Geometry check sheet. Reference: the model listing, model coordinates, mm. A direction names the side the tool comes from. Give positions to 0.01 mm unless a question says otherwise; leave off trailing zeros. Write each loop counter-clockwise with the first axis right and the second up, starting at its lowest first coordinate (ties: lowest second). Pieces come first, ordered by that corner, then holes. Notation, with made-up numbers: M 3.25,-6.75 L 48.25,-6.75 A34 cw 48.25,31.25 Z; hole C 54,-2.75 d6. An arc over 180 degrees is marked long. One line per item, written item: value. Start each with the question number.
1. Cross-section at B-B on z = 0. Record the cut outline in (x, y), then the cut area to 3 significant figures.
2. Gauge pin test, flat ends, axial feed: pin 1 (3 mm diameter, centred on y = 11, z = -22, fed in from +X); pin 2 (1 mm diameter, centred on y = 23, z = -7.5, fed in from +X); pin 3 (10 mm diameter, centred on y = 5, z = -12, fed in from -X). Record the tip position at first contact, or that the pin passes through.
3. Tool access check on faces 1 (the face through (-0.028, 17.255, 32.946)), 2 (the face through (-26.288, 21.514, 14.966)). Record the directions out of +Z, -Z, +X, -X, +Y, -Y that give a thin tool (end or side, any length) a straight path to the whole face; none if there is none.
4. Release check for a two-part mould opening along Z. For faces 3 (the face through (27.5, 21.5, 0.1)), 4 (the face through (0, 17, -33)), 5 (the face through (28, 35, 0)), 6 (the face through (0.18, 21.51, -30.25)) record: pulls with the +Z half, pulls with the -Z half, needs draft (parallel to the pull), parting line crosses it, or undercut.
5. Scan lines: line 1 (X direction, y = 30, z = 2.5); line 2 (Y direction, x = -10.5, z = -12); line 3 (Z direction, x = -21.5, y = 15.5). Record each from-to range of solid material in increasing order.
6. Cross-section at A-A on y = 22. Record the cut outline in (x, z) (3 decimals).
from build123d import *

# Parameters (mm, degrees)
BOSS_EXTRUDE1_DEPTH = 35
CUT_EXTRUDE2_DEPTH  = 36
BOSS_EXTRUDE2_DEPTH = 0.4
FILLET1_R           = 8


with BuildPart() as part:
    # Sketch1 → Boss-Extrude1 (new body)
    with BuildSketch(Plane(origin=(0, 0, 0), x_dir=(1, 0, 0), z_dir=(0, 1, 0))):
        with BuildLine():
            ThreePointArc((1.451818925, -34.068556857), (1.641248992, -34.346908706), (1.964225605, -34.442038138))
            ThreePointArc((1.964225605, -34.442038138), (26.591847487, -21.978073076), (34.198225299, 4.555174015))
            ThreePointArc((34.198225299, 4.555174015), (23.590291339, 25.176355888), (2.324135821, 34.423627607))
            ThreePointArc((2.324135821, 34.423627607), (1.751838249, 34.289058819), (1.354061739, 33.856153382))
            ThreePointArc((1.354061739, 33.856153382), (0, 33.001534515), (-1.354061739, 33.856153382))
            ThreePointArc((-1.354061739, 33.856153382), (-1.751838249, 34.289058819), (-2.324135821, 34.423627607))
            ThreePointArc((-2.324135821, 34.423627607), (-23.590291339, 25.176355888), (-34.198225299, 4.555174015))
            ThreePointArc((-34.198225299, 4.555174015), (-26.591847487, -21.978073076), (-1.964225605, -34.442038138))
            ThreePointArc((-1.964225605, -34.442038138), (-1.641248992, -34.346908706), (-1.451818925, -34.068556857))
            ThreePointArc((-1.451818925, -34.068556857), (0, -32.945679925), (1.451818925, -34.068556857))
        make_face()
        with BuildLine():
            Line((-2.417, 3.787737139), (0, 3.787737139))
            Line((0, 3.787737139), (2.417, 3.787737139))
            ThreePointArc((2.417, 3.787737139), (0, -4.489512172), (-2.417, 3.787737139))
        make_face(mode=Mode.SUBTRACT)
    extrude(amount=BOSS_EXTRUDE1_DEPTH)

    # Sketch2 → Cut-Extrude2 (cut, through all)
    with BuildSketch(Plane(origin=(0, 0, 0), x_dir=(1, 0, 0), z_dir=(0, 1, 0))):
        with BuildLine():
            ThreePointArc((-17.441608289, 24.715436478), (-26.197268464, 15.125), (-30.125, 2.747157622))
            ThreePointArc((-30.125, 2.747157622), (-27.5, 0), (-30.125, -2.747157622))
            ThreePointArc((-30.125, -2.747157622), (-26.197268464, -15.125), (-17.441608289, -24.715436478))
            ThreePointArc((-17.441608289, -24.715436478), (-13.75, -23.815698604), (-12.683391711, -27.4625941))
            ThreePointArc((-12.683391711, -27.4625941), (0, -30.25), (12.683391711, -27.4625941))
            ThreePointArc((12.683391711, -27.4625941), (13.75, -23.815698604), (17.441608289, -24.715436478))
            ThreePointArc((17.441608289, -24.715436478), (26.197268464, -15.125), (30.125, -2.747157622))
            ThreePointArc((30.125, -2.747157622), (27.5, 0), (30.125, 2.747157622))
            ThreePointArc((30.125, 2.747157622), (26.197268464, 15.125), (17.441608289, 24.715436478))
            ThreePointArc((17.441608289, 24.715436478), (13.75, 23.815698604), (12.683391711, 27.4625941))
            ThreePointArc((12.683391711, 27.4625941), (0, 30.25), (-12.683391711, 27.4625941))
            ThreePointArc((-12.683391711, 27.4625941), (-13.75, 23.815698604), (-17.441608289, 24.715436478))
        make_face()
    extrude(amount=CUT_EXTRUDE2_DEPTH, mode=Mode.SUBTRACT)

    # Sketch2<2> → Boss-Extrude2 (add)
    with BuildSketch(Plane(origin=(0, 0, 0), x_dir=(1, 0, 0), z_dir=(0, 1, 0))):
        with BuildLine():
            ThreePointArc((-17.441608289, 24.715436478), (-26.197268464, 15.125), (-30.125, 2.747157622))
            ThreePointArc((-30.125, 2.747157622), (-27.5, 0), (-30.125, -2.747157622))
            ThreePointArc((-30.125, -2.747157622), (-26.197268464, -15.125), (-17.441608289, -24.715436478))
            ThreePointArc((-17.441608289, -24.715436478), (-13.75, -23.815698604), (-12.683391711, -27.4625941))
            ThreePointArc((-12.683391711, -27.4625941), (0, -30.25), (12.683391711, -27.4625941))
            ThreePointArc((12.683391711, -27.4625941), (13.75, -23.815698604), (17.441608289, -24.715436478))
            ThreePointArc((17.441608289, -24.715436478), (26.197268464, -15.125), (30.125, -2.747157622))
            ThreePointArc((30.125, -2.747157622), (27.5, 0), (30.125, 2.747157622))
            ThreePointArc((30.125, 2.747157622), (26.197268464, 15.125), (17.441608289, 24.715436478))
            ThreePointArc((17.441608289, 24.715436478), (13.75, 23.815698604), (12.683391711, 27.4625941))
            ThreePointArc((12.683391711, 27.4625941), (0, 30.25), (-12.683391711, 27.4625941))
            ThreePointArc((-12.683391711, 27.4625941), (-13.75, 23.815698604), (-17.441608289, 24.715436478))
        make_face()
    extrude(amount=BOSS_EXTRUDE2_DEPTH)

    # Fillet1
    fillet1_edges = [part.edges().sort_by_distance(p)[0] for p in [
        (26.197268464, 0.4, 15.125),
        (27.5, 0.4, 0),
        (26.197268464, 0.4, -15.125),
        (13.75, 0.4, -23.815698604),
        (0, 0.4, -30.25),
        (-13.75, 0.4, -23.815698604),
        (-26.197268464, 0.4, -15.125),
        (-27.5, 0.4, 0),
        (-26.197268464, 0.4, 15.125),
        (-13.75, 0.4, 23.815698604),
        (0, 0.4, 30.25),
        (13.75, 0.4, 23.815698604),
    ]]
    fillet(fillet1_edges, radius=FILLET1_R)


solid = part.part
Report:
1. outline: M -34.5,0 L 34.5,0 L 34.5,35 L 27.5,35 L 27.5,8.4 A8 cw 19.5,0.4 L -19.5,0.4 A8 cw -27.5,8.4 L -27.5,35 L -34.5,35 Z
1. area: 539 mm^2
2. pin 1: stops at x = 27.75
2. pin 2: stops at x = 33.78
2. pin 3: stops at x = -33.78
3. face 1: +Z, +Y, -Y
3. face 2: +Y
4. face 3: undercut
4. face 4: pulls with the -Z half
4. face 5: needs draft
4. face 6: undercut
5. line 1: x = -34.41 to -29.1, 29.1 to 34.41
5. line 2: y = 0 to 0.4
5. line 3: z = -26.98 to -21.28, 21.28 to 26.98
6. outline: M -2.324,-34.424 A1 ccw -1.354,-33.856 A1.5 cw 1.354,-33.856 A1 ccw 2.324,-34.424 A34.5 ccw 1.964,34.442 A0.5 ccw 1.452,34.069 A1.5 cw -1.452,34.069 A0.5 ccw -1.964,34.442 A34.5 ccw Z; hole M -30.125,-2.747 A30.25 ccw -17.442,-24.715 A2.75 cw -12.683,-27.463 A30.25 ccw 12.683,-27.463 A2.75 cw 17.442,-24.715 A30.25 ccw 30.125,-2.747 A2.75 cw 30.125,2.747 A30.25 ccw 17.442,24.715 A2.75 cw 12.683,27.463 A30.25 ccw -12.683,27.463 A2.75 cw -17.442,24.715 A30.25 ccw -30.125,2.747 A2.75 cw Z
